```python
from build123d import *

# Parameters (mm, degrees)
EXTRUDE_1_DEPTH     = 80
CUT_EXTRUDE_1_DEPTH = 7.5
CUT_EXTRUDE_3_DEPTH = 102.118742081


with BuildPart() as part:
    # 草图1 → 凸台-拉伸1 (new body)
    with BuildSketch(Plane.XY):
        with BuildLine():
            Line((-7.5, -60), (-6, -60))
            Line((-6, -60), (-6, 0))
            ThreePointArc((-6, 0), (4.242640687, 4.242640687), (0, -6))
            Line((0, -6), (-5.5, -6))
            Line((-5.5, -6), (-5.5, -7.5))
            Line((-5.5, -7.5), (0, -7.5))
            ThreePointArc((0, -7.5), (5.303300859, 5.303300859), (-7.5, 0))
            Line((-7.5, 0), (-7.5, -60))
        make_face()
    extrude(amount=EXTRUDE_1_DEPTH)

    # 草图3 → 切除-拉伸1 (cut, symmetric)
    with BuildSketch(Plane(origin=(0, 0, 0), x_dir=(1, 0, 0), z_dir=(0, 1, 0))):
        Polygon((7.5, -40), (7.5, -32), (-7.5, -32), (-7.5, -48), (7.5, -48), align=None)
    extrude(amount=CUT_EXTRUDE_1_DEPTH, both=True, mode=Mode.SUBTRACT)

    # 草图5 → 切除-拉伸3 (cut, through all)
    with BuildSketch(Plane.ZY.offset(7.5)):
        Polygon((80, -60), (69.585166332, -11.440975615), (69.585166332, 7.476358761), (69.585166332, 9.692514451), (80, 9.692514451), (80, 7.5), align=None)
        Polygon((10.414833668, -11.440975615), (10.414833668, 7.476358761), (10.414833668, 9.692514451), (0, 9.692514451), (0, 7.5), (0, -60), align=None)
    extrude(amount=-CUT_EXTRUDE_3_DEPTH, mode=Mode.SUBTRACT)


solid = part.part
```
The listing builds one solid part. Answer for the finished solid, in the listing's coordinates (mm). A direction names the side the tool comes from. Coordinates: 2 decimals unless noted, no trailing zeros. Write each loop counter-clockwise with the first axis right and the second up, starting at its lowest first coordinate (ties: lowest second). Pieces come first, ordered by that corner, then holes. Notation, with made-up numbers: (41.25, -10) -> (84.25, -10) arc R14 ccw to (84.25, -4) -> close; hole circle Ø1 at (-20, 61). An arc over 180 degrees is marked (long way). Write each question's results on one line, items separated by ' | '. Start each with the question number.
1) A cutting plane is placed at C-C (y = -3.5). Determine the outline of the cut face in (x, z), then the cut area to 3 significant figures.
2) A cutting plane is placed at A-A (x = 4). Determine the outline of the cut face in (y, z).
3) Flat-ended cylindrical pins translate along their axes: pin 1 Ø6 at (x, z) = (-3.5, 24.5) entering from +Y; pin 2 Ø7.5 at (x, y) = (-1, -1) entering from +Z; pin 3 Ø1.6 at (x, z) = (-6.5, 40) entering from +Y; pin 4 Ø3 at (y, z) = (-37.5, 11.5) entering from +X. Find the tip coordinate at first contact, or state that the pin passes through.
4) Straight lines are drawn through the part: probe 1 along Y at (x, z) = (0, 52.5); probe 2 along X at (y, z) = (-22, 69); probe 3 along Y at (x, z) = (5.5, 29). For each, find the intervals that lie inside material, in ascending order.
5) A tool of negligible diameter and unlimited length cuts with its end or side. For faces 1 (the flat face through (-3, -6, 21)), 2 (the flat face through (-6.15, -1.93, 69.585)), 3 (the flat face through (-3, -7.5, 21)), 4 (the flat face through (-6.15, -1.08, 48)), from which of +Z, -Z, +X, -X, +Y, -Y can it reach the whole face along a straight path? Write none if from no direction.
6) A cutting plane is placed at B-B (z = 30). Determine the outline of the cut face in (x, y), then the cut area to 3 significant figures.
7) A cutting plane is placed at D-D (y = -50). Determine the outline of the cut face in (x, z).
8) For a pull along X with two mould halves and no side action, classify faces 5 (the cylindrical face through (4.1, 4.38, 21.06)), 6 (the cylindrical face through (5.5, 5.1, 21.1)), 7 (the flat face through (1.1, -6.1, 32)) as +X half, -X half, draft (parallel to the pull), parting line (faces both ways), or undercut.
Values follow:
1) outline: (-7.5, 10.41) -> (-6, 10.41) -> (-6, 32) -> (-7.5, 32) -> close; (-7.5, 48) -> (-6, 48) -> (-6, 69.59) -> (-7.5, 69.59) -> close; (4.87, 10.41) -> (6.63, 10.41) -> (6.63, 32) -> (4.87, 32) -> close; (4.87, 48) -> (6.63, 48) -> (6.63, 69.59) -> (4.87, 69.59) -> close | area: 141 mm²
2) outline: (-6.34, 10.41) -> (-4.47, 10.41) -> (-4.47, 32) -> (-6.34, 32) -> close; (-6.34, 48) -> (-4.47, 48) -> (-4.47, 69.59) -> (-6.34, 69.59) -> close; (4.47, 10.41) -> (6.34, 10.41) -> (6.34, 32) -> (4.47, 32) -> close; (4.47, 48) -> (6.34, 48) -> (6.34, 69.59) -> (4.47, 69.59) -> close
3) pin 1: y = 7.48 | pin 2: through | pin 3: y = -7.5 | pin 4: x = -6
4) probe 1: -7.5 to -6, 6 to 7.5 | probe 2: -7.5 to -6 | probe 3: -5.1 to -2.4, 2.4 to 5.1
5) face 1: +Z, -Z | face 2: +Z, +X, -X, +Y | face 3: +Z, -Z, +X, -Y | face 4: +X, -X, +Y
6) outline: (-7.5, -60) -> (-6, -60) -> (-6, 0) arc R6 cw (long way) to (0, -6) -> (-5.5, -6) -> (-5.5, -7.5) -> (0, -7.5) arc R7.5 ccw (long way) to (-7.5, 0) -> close | area: 146 mm²
7) outline: (-7.5, 2.14) -> (-6, 2.14) -> (-6, 77.86) -> (-7.5, 77.86) -> close
8) face 5: undercut | face 6: parting line | face 7: draft
